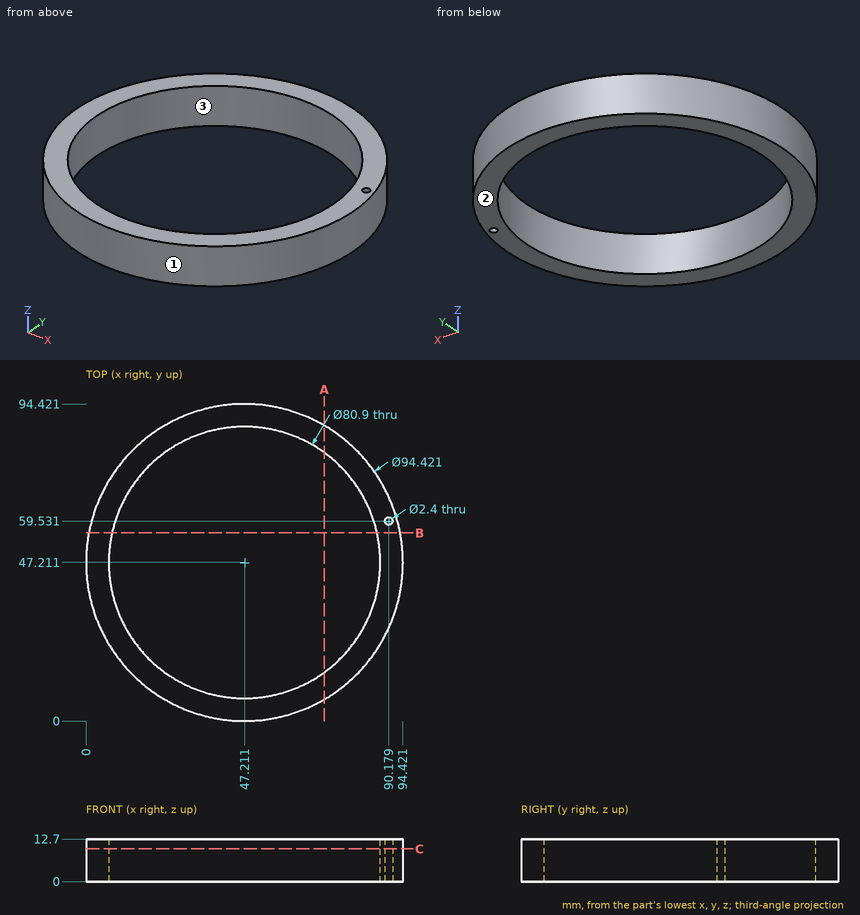
Could you check a few things on this drawing? It's one solid part, dimensions in mm from its lowest x, y, z. Coordinates: 2 decimals unless noted, no trailing zeros. Order: outer loops, then holes, each group sorted by start corner. A loop starts at its lowest first (then second) coordinate and runs counter-clockwise, first axis right, second up.
1. I need wall thicknesses on line 1 (X direction, y = 60, z = 7.75) (1 decimal); line 2 (X direction, y = 47, z = 11); line 3 (Y direction, x = 31.5, z = 8.5) (1 decimal). Which ranges of each line are inside material? Lowest first, please.
2. If we section it at A-A (x = 71): Please give me the cut outline in (y, z) (1 decimal), then the cut area to 3 significant figures.
3. If we section it at C-C (z = 9.75): Please give me the cut outline in (x, y).
4. If we section it at B-B (y = 56): Please give me the cut outline in (x, z) (1 decimal).
5. I'm going to push flat-ended pins straight in: pin 1 (8 mm diameter, centred on x = 68.5, y = 18, fed in from -Z); pin 2 (5 mm diameter, centred on y = 30, z = 6.5, fed in from -X); pin 3 (4 mm diameter, centred on x = 65.5, z = 1.5, fed in from +Y); pin 4 (1 mm diameter, centred on x = 71, z = 8, fed in from +Y). Where does each tip first touch, or does it pass through?
6. Thinking about a two-plate mould opening in Y: for the marked faces 1, 2 and 3, which applies, +Y half, -Y half, draft (parallel to the pull), parting line (faces both ways), or undercut?
Entries:
1. line 1: x = 1.8 to 8.8, 85.6 to 89.1, 91.3 to 92.7
1. line 2: x = 0 to 6.76, 87.66 to 94.42
1. line 3: y = 2.7 to 9.9, 84.5 to 91.7
2. outline: (6.4, 0) - (14.5, 0) - (14.5, 12.7) - (6.4, 12.7) - close; (79.9, 0) - (88, 0) - (88, 12.7) - (79.9, 12.7) - close
2. area: 205 mm2
3. outline: circle Ø94.42 at (47.21, 47.21); hole circle Ø80.9 at (47.21, 47.21); hole circle Ø2.4 at (90.18, 59.53)
4. outline: (0.8, 0) - (7.7, 0) - (7.7, 12.7) - (0.8, 12.7) - close; (86.7, 0) - (93.6, 0) - (93.6, 12.7) - (86.7, 12.7) - close
5. pin 1: passes through
5. pin 2: stops at x = 2.35
5. pin 3: stops at y = 91.52
5. pin 4: stops at y = 88.28
6. face 1: parting line
6. face 2: draft
6. face 3: undercut
